```python
from build123d import *

# Parameters (mm, degrees)
SKETCH_1_W                   = 40
SKETCH_1_H                   = 30
EXTRUDE_1_DEPTH              = 15
SKETCH_4_W                   = 35
SKETCH_4_H                   = 20
CUT_EXTRUDE_1_DEPTH          = 34.23784159
FILLET_1_R                   = 0.5
CUT_EXTRUDE_4_DEPTH          = 4
HOLE_WIZARD_M4_2_D           = 4.5
HOLE_WIZARD_M4_2_CBORE_D     = 8
HOLE_WIZARD_M4_2_CBORE_DEPTH = 4


with BuildPart() as part:
    # 草圖1 → 填料-伸長1 (new, symmetric)
    with BuildSketch(Plane.XY):
        Rectangle(SKETCH_1_W, SKETCH_1_H)
    extrude(amount=EXTRUDE_1_DEPTH, both=True)

    # 草圖4 → 除料-伸長1 (cut, through all)
    with BuildSketch(Plane(origin=(3.574759116, 0, 2.999579055), x_dir=(-0.6427876096865437, 0, 0.7660444431189745), z_dir=(0.7660444431189745, 0, 0.6427876096865437))):
        with Locations((-1.846418841, 0)):
            Rectangle(SKETCH_4_W, SKETCH_4_H)
    extrude(amount=CUT_EXTRUDE_1_DEPTH, mode=Mode.SUBTRACT)

    # 圓角1
    fillet_1_edges = [part.edges().sort_by_distance(p)[0] for p in [
        (16.010397438, 0, -11.820637592),
    ]]
    fillet(fillet_1_edges, radius=FILLET_1_R)

    # 草圖7 → 除料-伸長4 (cut)
    with BuildSketch(Plane(origin=(12.435638322, 0, -14.820216647), x_dir=(0.7660444431189746, 0, 0.6427876096865437), z_dir=(-0.6427876096865437, 0, 0.7660444431189746))):
        with BuildLine():
            Line((9.874572873, -2.236067977), (9.874572873, 2.236067977))
            ThreePointArc((9.874572873, 2.236067977), (8.874572873, 0), (9.874572873, -2.236067977))
        make_face()
    extrude(amount=-CUT_EXTRUDE_4_DEPTH, mode=Mode.SUBTRACT)

    # M4 凹頭蓋螺釘的柱孔2 (through all)
    with Locations(Plane.XY.offset(15)):
        with Locations((-15, 10), (-15, -10)):
            CounterBoreHole(HOLE_WIZARD_M4_2_D / 2, HOLE_WIZARD_M4_2_CBORE_D / 2, HOLE_WIZARD_M4_2_CBORE_DEPTH)


solid = part.part
```
Check sheet for the modelled part. Datum: model origin and axes. Units: mm. A direction names the side the tool comes from. Round coordinates to 2 decimals unless told otherwise and drop trailing zeros. Order: outer loops, then holes, each group sorted by start corner. A loop starts at its lowest first (then second) coordinate and runs counter-clockwise, first axis right, second up. Notation, with made-up numbers: (69.5, 26.25) -> (81.5, 26.25) arc R15 cw to (81.5, 54.25) -> close; hole circle Ø7 at (25, -39). An arc over 180 degrees is marked (long way). One line per item, written item: value. Start each with the question number.
Q1. Cross-section at A-A (x = -15). Record the boundary of the cut face in (y, z).
Q2. Cross-section at B-B (z = 10). Record the boundary of the cut face in (x, y).
Q3. Cross-section at D-D (z = -8). Record the boundary of the cut face in (x, y), and give its area (3 significant figures).
Q4. Set-up check for faces 5 (the face through (-13, 8, 11)), 6 (the face through (-16.21, 11.897, -2.182)): record each of +Z, -Z, +X, -X, +Y, -Y from which the full face is reachable in a straight line by a thin tool's end or side.
Q5. Gauge pin test, flat ends, axial feed: pin 1 Ø9 at (x, y) = (-17, -8.5) entering from +Z; pin 2 Ø2.5 at (x, y) = (-15, 10) entering from -Z; pin 3 Ø5 at (x, y) = (-15, 10) entering from +Z; pin 4 Ø3 at (x, y) = (10, -1.5) entering from +Z. Record the tip position at first contact, or that the pin passes through.
Q6. Thickness scan on line 1 (Y direction, x = -15, z = -5.25); line 2 (Y direction, x = -15, z = 13.9); line 3 (Y direction, x = 16, z = -6.5). Record the ranges inside material, lowest first.
Q7. Mould release check, pull along X, two halves, no side actions. Record for faces 1 (the face through (18.17, 0.14, -10.01)), 2 (the face through (-13, -12, 11)), 3 (the face through (0, 0, -15)), 4 (the face through (19.573, 0.035, -9.519)): pulls with the +X half, pulls with the -X half, needs draft (parallel to the pull), parting line crosses it, or undercut.
Completed:
1. outline: (-15, -15) -> (-12.25, -15) -> (-12.25, 11) -> (-14, 11) -> (-14, 15) -> (-15, 15) -> close; (-7.75, -15) -> (7.75, -15) -> (7.75, 11) -> (6, 11) -> (6, 15) -> (-6, 15) -> (-6, 11) -> (-7.75, 11) -> close; (12.25, -15) -> (15, -15) -> (15, 15) -> (14, 15) -> (14, 11) -> (12.25, 11) -> close
2. outline: (-20, -15) -> (20, -15) -> (20, -10) -> (-2.3, -10) -> (-2.3, 10) -> (20, 10) -> (20, 15) -> (-20, 15) -> close; hole circle Ø4.5 at (-15, -10); hole circle Ø4.5 at (-15, 10)
3. outline: (-20, -15) -> (20, -15) -> (20, -10) -> (12.8, -10) -> (12.8, 10) -> (20, 10) -> (20, 15) -> (-20, 15) -> close; hole circle Ø4.5 at (-15, -10); hole circle Ø4.5 at (-15, 10)
3. area: 1,020 mm²
4. face 5: +Z
4. face 6: +Z, -Z
5. pin 1: stops at z = 15
5. pin 2: passes through
5. pin 3: stops at z = 11
5. pin 4: stops at z = -2.87
6. line 1: y = -15 to -12.25, -7.75 to 7.75, 12.25 to 15
6. line 2: y = -15 to -14, -6 to 6, 14 to 15
6. line 3: y = -15 to -10, 10 to 15
7. face 1: undercut
7. face 2: undercut
7. face 3: needs draft
7. face 4: pulls with the +X half
